Can you work these out from the model? Positions are in its coordinate system, mm. Face numbers are marked on the shaded views. Round coordinates to 2 decimals unless told otherwise and drop trailing zeros. Write each loop counter-clockwise with the first axis right and the second up, starting at its lowest first coordinate (ties: lowest second). Pieces come first, ordered by that corner, then holes. Notation, with made-up numbers: M -2.5,6.5 L 53.5,6.5 A31 cw 53.5,41.5 Z; hole C -0.5,70.25 d10. An arc over 180 degrees is marked long. Use one line per item in the form item = value. Start each with the question number.
```python
from build123d import *

# Parameters (mm, degrees)
SKETCH1_R               = 5.225
SKETCH1_R_2             = 2.5
BOSS_EXTRUDE1_DEPTH     = 5.25
SKETCH2_R               = 1.5
CUT_EXTRUDE1_DEPTH      = 5.225
CUT_EXTRUDE2_DEPTH      = 10.064422392
CUT_EXTRUDE2_DEPTH_BACK = 10.064422392
SKETCH4_R               = 9
FILLET1_R               = 0.25
CHAMFER1_SIZE           = 0.25


with BuildPart() as part:
    # Sketch1 → Boss-Extrude1 (new, symmetric)
    with BuildSketch(Plane(origin=(0, 0, 0), x_dir=(1, 0, 0), z_dir=(0, 1, 0))):
        with Locations(Location((0, 0, 0), (0, 0, 90))):
            Circle(SKETCH1_R)
        with Locations(Location((0, 0, 0), (0, 0, 90))):
            Circle(SKETCH1_R_2, mode=Mode.SUBTRACT)
    extrude(amount=BOSS_EXTRUDE1_DEPTH, both=True)

    # Sketch2 → Cut-Extrude1 (cut, symmetric)
    with BuildSketch(Plane.XY):
        Circle(SKETCH2_R)
    extrude(amount=CUT_EXTRUDE1_DEPTH, both=True, mode=Mode.SUBTRACT)

    # Sketch4 → Cut-Extrude2 (cut, two sides: drawn at the far end of the back side and taken through both)
    with BuildSketch(Plane(origin=(0, 0, 0), x_dir=(0, 0, -1), z_dir=(1, 0, 0)).offset(-CUT_EXTRUDE2_DEPTH_BACK)):
        with Locations((-14, 0)):
            Circle(SKETCH4_R)
    extrude(amount=CUT_EXTRUDE2_DEPTH + CUT_EXTRUDE2_DEPTH_BACK, mode=Mode.SUBTRACT)

    # Fillet1
    fillet1_edges = [part.edges().sort_by_distance(p)[0] for p in [
        (0, -5.25, 5.225),
        (0, 5.25, 5.225),
    ]]
    fillet(fillet1_edges, radius=FILLET1_R)

    # Chamfer1
    chamfer1_edges = [part.edges().sort_by_distance(p)[0] for p in [
        (0, 5.25, 2.5),
    ]]
    chamfer(chamfer1_edges, length=CHAMFER1_SIZE)


solid = part.part
```
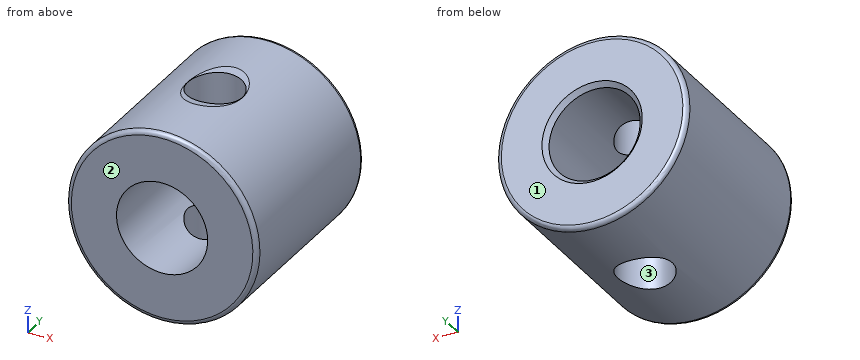
1. If we section it at B-B (y = 4.75): List the corners of the cut face in (x, z) for me (3 decimals).
2. Will these pins go through, and if not, where does the flat tip stop? pin 1 (3 mm diameter, centred on x = -3.5, y = -0.5, fed in from -Z); pin 2 (1 mm diameter, centred on y = 4, z = 2.5, fed in from -X); pin 3 (2 mm diameter, centred on y = 4, z = 3.5, fed in from +X).
3. Please list where these lines run through material, in increasing order: line 1 along Y through (x, z) = (0, 3.8); line 2 along X through (y, z) = (1.75, 0) (3 decimals); line 3 along X through (y, z) = (0, 4.35).
4. If we section it at C-C (x = 1): State how many separate pieces and enclosed holes the cut face has, and give its area (3 significant figures).
5. If we section it at A-A (z = 0): List the corners of the cut face in (x, y) for me (3 decimals).
6. If we mould it in two halves opening along Y, with no side actions, what happens to the marked faces 1, 2 and 3? For each: pulls with the +Y half, pulls with the -Y half, needs draft (parallel to the pull), parting line crosses it, or undercut.
Model answer:
q1.outline = C 0,0 d10.45; hole C 0,0 d5
q2.pin_1 = -4.83
q2.pin_2 = -4.83
q2.pin_3 = 4.59
q3.line_1 = -5.25 to -1.5, 1.5 to 5.25
q3.line_2 = -5.225 to -2.5, 2.5 to 5.225
q3.line_3 = -2.89 to -1.5, 1.5 to 2.89
q4.separate_pieces = 4
q4.enclosed_holes = 0
q4.area = 46.7 mm2
q5.outline = M -5.225,-5 A0.25 ccw -4.975,-5.25 L -2.5,-5.25 L -2.5,5 L -2.75,5.25 L -4.975,5.25 A0.25 ccw -5.225,5 Z; M 2.5,-5.25 L 4.975,-5.25 A0.25 ccw 5.225,-5 L 5.225,5 A0.25 ccw 4.975,5.25 L 2.75,5.25 L 2.5,5 Z
q6.face_1 = pulls with the +Y half
q6.face_2 = pulls with the -Y half
q6.face_3 = undercut
